Check sheet for the modelled part. Datum: model origin and axes. Units: mm. A direction names the side the tool comes from. Coordinates: 2 decimals unless noted, no trailing zeros. Write each loop counter-clockwise with the first axis right and the second up, starting at its lowest first coordinate (ties: lowest second). Pieces come first, ordered by that corner, then holes. Notation, with made-up numbers: (13, -2.5) -> (56, -2.5) arc R18 ccw to (56, 8.5) -> close; hole circle Ø2 at (21.5, 5.5). An arc over 180 degrees is marked (long way). Put each result on its own line as item: value.
```python
from build123d import *

# Parameters (mm, degrees)
F1_DEPTH = 20
F2_R     = 6
F3_DEPTH = 10


with BuildPart() as f1:
    # F0 (on Right) → F1 (new body)
    with BuildSketch(Plane.YZ):
        Polygon((12.5, -14.775001), (-22.5, -14.775001), (-22.5, -32.975001), (22.5, -32.975001), (22.5, -22.975001), align=None)
    extrude(amount=-F1_DEPTH)

    # F2 (on face) → F3 (join)
    with BuildSketch(Plane(origin=(0, 0, -32.975001), x_dir=(1, 0, 0), z_dir=(0, 0, -1))):
        with Locations((-10, -12.5)):
            Circle(F2_R)
    extrude(amount=F3_DEPTH)


solid = f1.part
```
Q1. Depth check by flat-ended pin: P1, Ø5, axis at y = -1, z = -31.5, coming from the +X side; P2, Ø6, axis at x = -12.5, z = -36.5, coming from the -Y side; P3, Ø1.5, axis at x = -6.5, y = -12.5, coming from the -Z side (3 decimals); P4, Ø4, axis at y = 9.5, z = -39.5, coming from the -X side. Enter the tip coordinate at first touch or a pass-through.
Recorded:
P1: stops at x = 0
P2: stops at y = 6.5
P3: stops at z = -32.975
P4: stops at x = -15.92
Q2. Material ranges on line 1 along Z through (x, y) = (-18.25, -19.5) (3 decimals); line 2 along Z through (x, y) = (-9.5, 21) (3 decimals); line 3 along X through (y, z) = (12.5, -40), recorded low to high.
Recorded:
line 1: z = -32.975 to -14.775
line 2: z = -32.975 to -21.745
line 3: x = -16 to -4
Q3. Cross-section at B-B (y = 7.5). Record the cut outline in (x, z) (3 decimals), plus the area to 3 significant figures.
Recorded:
outline: (-20, -32.975) -> (-13.317, -32.975) -> (-13.317, -42.975) -> (-6.683, -42.975) -> (-6.683, -32.975) -> (0, -32.975) -> (0, -14.775) -> (-20, -14.775) -> close
area: 430 mm2
Q4. Cross-section at D-D (x = -2). Record the cut outline in (y, z) (3 decimals).
Recorded:
outline: (-22.5, -32.975) -> (22.5, -32.975) -> (22.5, -22.975) -> (12.5, -14.775) -> (-22.5, -14.775) -> close
Q5. Cross-section at C-C (z = -39.75). Record the cut outline in (x, y), plus the area to 3 significant figures.
Recorded:
outline: circle Ø12 at (-10, 12.5)
area: 113 mm2
Q6. Tool access check on faces 1 (the flat face through (-10, -22.5, -24)), 2 (the cylindrical face through (-6.774, 7.441, -37.905)). Record the directions out of +Z, -Z, +X, -X, +Y, -Y that give a thin tool (end or side, any length) a straight path to the whole face; none if there is none.
Recorded:
face 1: +Z, -Z, +X, -X, -Y
face 2: -Z
Q7. Cross-section at A-A (x = -10). Record the cut outline in (y, z) (3 decimals).
Recorded:
outline: (-22.5, -32.975) -> (6.5, -32.975) -> (6.5, -42.975) -> (18.5, -42.975) -> (18.5, -32.975) -> (22.5, -32.975) -> (22.5, -22.975) -> (12.5, -14.775) -> (-22.5, -14.775) -> close
